Autodesk Inventor part; units mm, degrees
ref_plane "Work Plane1" through (-17, 2, 0) normal (0, 0, 1) x (1, 0, 0)
ref_plane "YZ Plane" through (0, 0, 0) normal (1, 0, 0) x (0, 1, 0)
ref_plane "XZ Plane" through (0, 0, 0) normal (0, 1, 0) x (-1, 0, 0)
sketch "Sketch1" plane through (0, 0, 0) normal (0, 1, 0) x (-1, 0, 0)
  line L0 (-17, 25) -> (17, 25)
  line L1 (17, 25) -> (17, -25)
  line L2 (17, -25) -> (-17, -25)
  line L3 (-17, -25) -> (-17, 25)
  line L4 (-17, 25) -> (17, -25) construction
  line L5 (17, 25) -> (-17, -25) construction
  point P0 (0, 0)
  dimension "d0" = 34
  dimension "d1" = 50
extrude "Extrusion1" add sketch "Sketch1" along normal blind 2
sketch "Sketch2" plane through (0, 2, 0) normal (0, 1, 0) x (1, 0, 0)
  line L0 (17, 25) -> (-17, 25)
  line L1 (0, 25) -> (0, 18.3)
  line L2 (0, 18.3) -> (-1.27, 18.3)
  line L3 (-1.27, 18.3) -> (-3.81, 18.3)
  line L4 (-3.81, 18.3) -> (-6.35, 18.3)
  line L5 (-6.35, 18.3) -> (-8.89, 18.3)
  line L6 (-8.89, 18.3) -> (-11.43, 18.3)
  line L7 (0, 18.3) -> (1.27, 18.3)
  line L8 (1.27, 18.3) -> (3.81, 18.3)
  line L9 (3.81, 18.3) -> (6.35, 18.3)
  line L10 (6.35, 18.3) -> (8.89, 18.3)
  line L11 (8.89, 18.3) -> (11.43, 18.3)
  circle A0 centre (-11.43, 18.3) radius 0.5
  circle A1 centre (-8.89, 18.3) radius 0.5
  circle A2 centre (-6.35, 18.3) radius 0.5
  circle A3 centre (-3.81, 18.3) radius 0.5
  circle A4 centre (-1.27, 18.3) radius 0.5
  circle A5 centre (1.27, 18.3) radius 0.5
  circle A6 centre (3.81, 18.3) radius 0.5
  circle A7 centre (6.35, 18.3) radius 0.5
  circle A8 centre (8.89, 18.3) radius 0.5
  circle A9 centre (11.43, 18.3) radius 0.5
  point P0 (0, 0)
  dimension "d4" = 6.7
  dimension "d5" = 1.27
  dimension "d6" = 2.54
  dimension "d7" = 2.54
  dimension "d8" = 2.54
  dimension "d9" = 2.54
  dimension "d10" = 1.27
  dimension "d11" = 2.54
  dimension "d12" = 2.54
  dimension "d13" = 2.54
  dimension "d14" = 2.54
  dimension "d15" = 1
  dimension "d16" = 1
  dimension "d17" = 1
  dimension "d18" = 1
  dimension "d19" = 1
  dimension "d20" = 1
  dimension "d21" = 1
  dimension "d22" = 1
  dimension "d23" = 1
  dimension "d24" = 1
extrude "Extrusion2" cut sketch "Sketch2" against normal up to next
ref_plane "Work Plane1" through (-17, 2, 0) normal (0, 0, 1) x (1, 0, 0)
mirror "Mirror1" about plane through (-17, 2, 0) normal (0, 0, 1) of "Extrusion2"
properties part number "pcb"
Source: CAD feature listing. Evaluate the final solid. Frame: model axes, mm. Give positions to 0.01 mm unless a question says otherwise; leave off trailing zeros. Loops run counter-clockwise (first coordinate to the right, second up) from the corner with the lowest first, then second, coordinate; pieces in that order, holes last. Notation, with made-up numbers: (-37, 40.25) - (-17, 40.25) arc R16 ccw to (-17, 62.25) - close; hole circle Ø9 at (-24.75, -32). An arc over 180 degrees is marked (long way). Use CSV: the item, a comma, the result in double quotes.
1) Cut plane A-A (x = -6.35). Output: boundary loops of the cut face in (y, z).
Worked out:
outline,"(0, -25) - (2, -25) - (2, -18.8) - (0, -18.8) - close; (0, -17.8) - (2, -17.8) - (2, 17.8) - (0, 17.8) - close; (0, 18.8) - (2, 18.8) - (2, 25) - (0, 25) - close"
2) Mould query, pull axis Z, two halves, no side actions, for faces 1 (the flat face through (0, 1, 25)), 2 (the flat face through (-17, 1, 0)), 3 (the cylindrical face through (3.745, 1.014, -18.796)). Classes: +Z half, -Z half, draft (parallel to the pull), parting line (faces both ways), or undercut.
Worked out:
face 1,"+Z half"
face 2,"draft"
face 3,"undercut"
3) Line query: line 1 (Z direction, x = 11.5, y = 0.55); line 2 (Z direction, x = -11, y = 1.6). Output: solid intervals per line, ascending.
Worked out:
line 1,"z = -25 to -18.8, -17.8 to 17.8, 18.8 to 25"
line 2,"z = -25 to -18.56, -18.04 to 18.04, 18.56 to 25"
